Here's how the part is built. I have some questions about the finished solid (model axes, mm). Coordinates: 2 decimals unless noted, no trailing zeros. Loops run counter-clockwise (first coordinate to the right, second up) from the corner with the lowest first, then second, coordinate; pieces in that order, holes last. Notation, with made-up numbers: (-25.75, -17.75) - (-7.75, -17.75) arc R22 ccw to (-7.75, -0.75) - close; hole circle Ø9 at (23.5, 73). An arc over 180 degrees is marked (long way). Use a Markdown table: item, result.
Autodesk Inventor part; units mm, degrees
ref_plane "YZ Plane" through (0, 0, 0) normal (1, 0, 0) x (0, 1, 0)
ref_plane "XZ Plane" through (0, 0, 0) normal (0, 1, 0) x (-1, 0, 0)
ref_plane "XY Plane" through (0, 0, 0) normal (0, 0, 1) x (1, 0, 0)
sketch "スケッチ1" plane through (0, 0, 0) normal (0, 0, 1) x (1, 0, 0)
  circle A0 centre (152.1225, -73.6752) radius 4
  line L0 (206.0478, 0.7) -> (205.7783, 0.7)
  circle A1 centre (152.1225, -73.6752) radius 4
  line L1 (206.0478, 0.7) -> (205.7783, 0.7)
  circle A2 centre (171.8792, -18.7507) radius 14
  circle A3 centre (-152.1225, 73.6752) radius 4
  line L2 (-206.0478, -0.7) -> (-205.7783, -0.7)
  circle A4 centre (-152.1225, 73.6752) radius 4
  line L3 (-206.0478, -0.7) -> (-205.7783, -0.7)
  circle A5 centre (-171.8792, 18.7507) radius 14
  line L4 (-152.1225, 73.6752) -> (-155.4555, 75.8868)
  line L5 (-155.4555, 75.8868) -> (-205.8083, 0)
  circle A6 centre (152.1225, -73.6752) radius 4
  line L6 (206.0478, 0.7) -> (205.7783, 0.7)
  circle A7 centre (171.8792, -18.7507) radius 14
  line L7 (250, 0) -> (156.4849, 0)
  line L8 (-250, 0) -> (-156.4849, 0)
  line L9 (-205.8083, -0.7) -> (-205.8083, 0)
  line L10 (-206.5583, -0.7) -> (-206.5583, 0.2262)
  line L11 (-206.5583, 0.2262) -> (-155.6658, 76.9264)
  line L12 (-155.6658, 76.9264) -> (-151.7078, 74.3002) construction
  line L13 (-155.4555, 75.8868) -> (-156.0804, 76.3015)
  line L14 (-205.8083, 0) -> (-206.4332, 0.4147)
  line L15 (-203.6688, 4.5809) -> (-203.0438, 4.1663)
  line L16 (-158.2199, 71.7205) -> (-158.8449, 72.1352)
  point P0 (0, 0)
  point P1 (205.8083, 0.7)
  point P2 (205.8083, 0.7)
  point P3 (205.8083, 0.7)
  dimension "d2" = 360
  dimension "d6" = 360
  dimension "d8" = 0.75
  dimension "d11" = 5
  dimension "d12" = 5
  dimension "d27" = 56.435
extrude "押し出し1" add sketch "スケッチ1" along normal blind 78.6 contours L5 L16 L11 L13 | L5 L15 L11 L16 | L5 L14 L11 L15
sketch "スケッチ2" plane through (-206.4332, 0.4147, 0) normal (-0.8333, 0.5529, 0) x (0, 0, 1)
  line L0 (0, 91.0725) -> (0, 0)
  line L1 (0, 0) -> (78.6, 0)
  line L2 (78.6, 91.0725) -> (78.6, 0)
  line L3 (0, 91.0725) -> (78.6, 91.0725)
  line L4 (0, 86.0725) -> (78.6, 86.0725)
  line L5 (0, 5) -> (78.6, 5)
  line L6 (39.3, 91.0725) -> (39.3, 0)
  circle A0 centre (22.3, 5) radius 1.5
  circle A1 centre (56.3, 5) radius 1.5
  circle A2 centre (22.3, 86.0725) radius 1.5
  circle A3 centre (56.3, 86.0725) radius 1.5
  point P0 (0, 113.7886)
  dimension "d13" = 5
  dimension "d14" = 5
  dimension "d15" = 39.3
  dimension "d16" = 39.3
  dimension "d17" = 3
  dimension "d18" = 3
  dimension "d19" = 3
  dimension "d20" = 3
  dimension "d21" = 17
  dimension "d22" = 17
  dimension "d23" = 17
  dimension "d24" = 17
extrude "押し出し2" cut sketch "スケッチ2" against normal blind 10 contours A2 L4 | L4 A2 | A0 L5 | L5 A0 | A3 L4 | L4 A3 | A1 L5 | L5 A1
properties part number "モーターガード" material "ポリプロピレン"
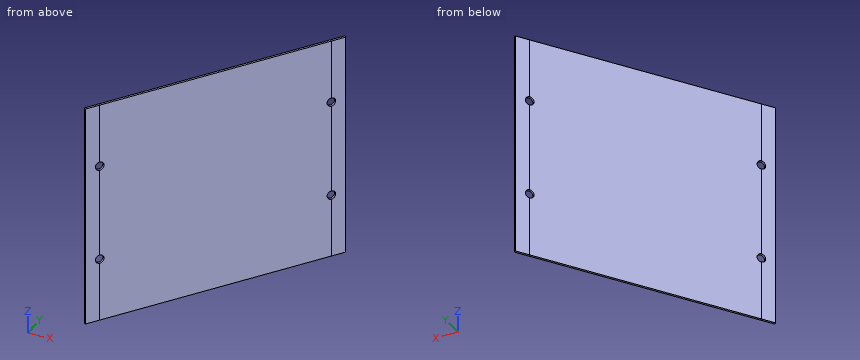
Q1. Please list where these lines run through material, in increasing order: L1, parallel to Y at x = -186.5, z = 50.5; L2, parallel to X at y = 13.5, z = 26; L3, parallel to Y at x = -179.5, z = 9.5. Write a range as from..to.
Check values:
| item | result |
|---|---|
| L1 | 29.1..30.46 |
| L2 | -197.75..-196.85 |
| L3 | 39.65..41.01 |
Q2. I want a section at B-B, the plane y = 53. Write out the boundary of the cut face in (x, z), then the cut area to 3 significant figures.
Check values:
| item | result |
|---|---|
| outline | (-171.54, 0) - (-170.64, 0) - (-170.64, 78.6) - (-171.54, 78.6) - close |
| area | 70.8 mm^2 |
Q3. Will these pins go through, and if not, where does the flat tip stop? P1, Ø2, axis at x = -167, z = 69, coming from the +Y side; P2, Ø4, axis at y = 35.5, z = 67.5, coming from the -X side; P3, Ø4, axis at x = -173, z = 49, coming from the +Y side.
Check values:
| item | result |
|---|---|
| P1 | y = 61.35 |
| P2 | x = -184.48 |
| P3 | y = 53.82 |
Q4. I want a section at C-C, the plane x = -183.5. Write out the boundary of the cut face in (y, z).
Check values:
| item | result |
|---|---|
| outline | (33.62, 0) - (34.98, 0) - (34.98, 78.6) - (33.62, 78.6) - close |
Q5. I want a section at A-A, the plane z = 33. Write out the boundary of the cut face in (x, y).
Check values:
| item | result |
|---|---|
| outline | (-206.43, 0.41) - (-205.81, 0) - (-155.46, 75.89) - (-156.08, 76.3) - close |
